```python
from build123d import *

# Parameters (mm, degrees)
F0_R     = 1.85
F0_R_2   = 4
F0_W     = 10.16
F0_H     = 6.35
F0_W_2   = 12.7
F0_W_3   = 6.35
F0_H_2   = 15.24
F0_H_3   = 8.021719
F1_DEPTH = 6.35


with BuildPart() as f1:
    # F0 (on Top) → F1 (new body)
    with BuildSketch(Plane.XY):
        with BuildLine():
            Line((-60.850162, -6.604), (-60.850162, 0))
            Line((-60.850162, 0), (-54.533258, 0))
            Line((-54.533258, 0), (-54.533258, 203.2))
            add(Edge.make_bspline(
                [(-54.533258, 203.2), (-23.033295, 215.9), (23.033295, 215.9), (54.533258, 203.2)],
                knots=[0, 0, 0, 0, 109.066515, 109.066515, 109.066515, 109.066515], degree=3))
            Line((54.533258, 203.2), (54.533258, 0))
            Line((54.533258, 0), (60.850162, 0))
            Line((60.850162, 0), (60.850162, -6.604))
            Line((60.850162, -6.604), (89.198314, -6.604))
            Line((89.198314, -6.604), (89.198314, 0))
            Line((89.198314, 0), (94.278314, 0))
            Line((94.278314, 0), (94.278314, 38.1))
            Line((94.278314, 38.1), (100.882314, 38.1))
            Line((100.882314, 38.1), (100.882314, 88.9))
            Line((100.882314, 88.9), (94.278314, 88.9))
            Line((94.278314, 88.9), (94.278314, 114.3))
            Line((94.278314, 114.3), (100.882314, 114.3))
            Line((100.882314, 114.3), (100.882314, 165.1))
            Line((100.882314, 165.1), (94.278314, 165.1))
            Line((94.278314, 165.1), (94.278314, 203.2))
            Line((94.278314, 203.2), (58.854451, 279.166719))
            Line((58.854451, 279.166719), (9.525, 279.166719))
            Line((9.525, 279.166719), (9.525, 263.525))
            Line((9.525, 263.525), (20.955, 263.525))
            Line((20.955, 263.525), (20.955, 248.285))
            Line((20.955, 248.285), (9.525, 248.285))
            Line((9.525, 248.285), (9.525, 241.066719))
            Line((9.525, 241.066719), (-9.525, 241.066719))
            Line((-9.525, 241.066719), (-9.525, 279.166719))
            Line((-9.525, 279.166719), (-58.854451, 279.166719))
            Line((-58.854451, 279.166719), (-94.278314, 203.2))
            Line((-94.278314, 203.2), (-94.278314, 165.1))
            Line((-94.278314, 165.1), (-100.882314, 165.1))
            Line((-100.882314, 165.1), (-100.882314, 114.3))
            Line((-100.882314, 114.3), (-94.278314, 114.3))
            Line((-94.278314, 114.3), (-94.278314, 88.9))
            Line((-94.278314, 88.9), (-100.882314, 88.9))
            Line((-100.882314, 88.9), (-100.882314, 38.1))
            Line((-100.882314, 38.1), (-94.278314, 38.1))
            Line((-94.278314, 38.1), (-94.278314, 0))
            Line((-94.278314, 0), (-89.198314, 0))
            Line((-89.198314, 0), (-89.198314, -6.604))
            Line((-89.198314, -6.604), (-60.850162, -6.604))
        make_face()
        with Locations((-80.681092, 9.743146)):
            Circle(F0_R, mode=Mode.SUBTRACT)
        with Locations((-80.681092, 21.056854)):
            Circle(F0_R, mode=Mode.SUBTRACT)
        with Locations((-69.367384, 9.743146)):
            Circle(F0_R, mode=Mode.SUBTRACT)
        with Locations((-75.024238, 15.4)):
            Circle(F0_R_2, mode=Mode.SUBTRACT)
        with Locations((-69.367384, 21.056854)):
            Circle(F0_R, mode=Mode.SUBTRACT)
        with Locations((-75.024238, 63.5)):
            Rectangle(F0_W, F0_H, mode=Mode.SUBTRACT)
        with Locations((69.367384, 9.743146)):
            Circle(F0_R, mode=Mode.SUBTRACT)
        with Locations((75.024238, 15.4)):
            Circle(F0_R_2, mode=Mode.SUBTRACT)
        with Locations((69.367384, 21.056854)):
            Circle(F0_R, mode=Mode.SUBTRACT)
        with Locations((80.681092, 9.743146)):
            Circle(F0_R, mode=Mode.SUBTRACT)
        with Locations((80.681092, 21.056854)):
            Circle(F0_R, mode=Mode.SUBTRACT)
        with Locations((75.024238, 63.5)):
            Rectangle(F0_W, F0_H, mode=Mode.SUBTRACT)
        with Locations((-75.024238, 139.7)):
            Rectangle(F0_W, F0_H, mode=Mode.SUBTRACT)
        with Locations((-74.405786, 200.025)):
            Rectangle(F0_W_2, F0_H, mode=Mode.SUBTRACT)
        with Locations((-17.78, 227.960319)):
            Rectangle(F0_W_3, F0_H_2, mode=Mode.SUBTRACT)
        with Locations((-17.78, 255.905)):
            Rectangle(F0_W_3, F0_H_2, mode=Mode.SUBTRACT)
        with Locations((75.024238, 139.7)):
            Rectangle(F0_W, F0_H, mode=Mode.SUBTRACT)
        with Locations((74.405786, 200.025)):
            Rectangle(F0_W_2, F0_H, mode=Mode.SUBTRACT)
        with Locations((0, 226.895859)):
            Rectangle(F0_W_3, F0_H_3, mode=Mode.SUBTRACT)
        with Locations((17.78, 227.960319)):
            Rectangle(F0_W_3, F0_H_2, mode=Mode.SUBTRACT)
    extrude(amount=F1_DEPTH)


solid = f1.part
```
Input: part model. Units: mm. Frame: model coordinates. A direction names the side the tool comes from. Round coordinates to 2 decimals unless told otherwise and drop trailing zeros. Order: outer loops, then holes, each group sorted by start corner. A loop starts at its lowest first (then second) coordinate and runs counter-clockwise, first axis right, second up. Notation, with made-up numbers: (18, 68) - (62, 68) arc R21 ccw to (62, 95) - close; hole circle Ø1 at (14, 18). An arc over 180 degrees is marked (long way). Answer in a Markdown table with one row per item.
Item 1: Section query B-B (y = 15.4). Return the cut outline in (x, z), then the cut area to 3 significant figures.
Model answer:
| item | result |
|---|---|
| outline | (-94.28, 0) - (-79.02, 0) - (-79.02, 6.35) - (-94.28, 6.35) - close; (-71.02, 0) - (-54.53, 0) - (-54.53, 6.35) - (-71.02, 6.35) - close; (54.53, 0) - (71.02, 0) - (71.02, 6.35) - (54.53, 6.35) - close; (79.02, 0) - (94.28, 0) - (94.28, 6.35) - (79.02, 6.35) - close |
| area | 403 mm² |
Item 2: Section query A-A (y = 105). Return the cut outline in (x, z).
Model answer:
| item | result |
|---|---|
| outline | (-94.28, 0) - (-54.53, 0) - (-54.53, 6.35) - (-94.28, 6.35) - close; (54.53, 0) - (94.28, 0) - (94.28, 6.35) - (54.53, 6.35) - close |
Item 3: Section query C-C (y = 149.5). Return the cut outline in (x, z).
Model answer:
| item | result |
|---|---|
| outline | (-100.88, 0) - (-54.53, 0) - (-54.53, 6.35) - (-100.88, 6.35) - close; (54.53, 0) - (100.88, 0) - (100.88, 6.35) - (54.53, 6.35) - close |
Item 4: Reachability of faces 4 (the flat face through (89.198, -3, 3)), 5 (the flat face through (75, 60.325, 3)), 6 (the flat face through (60.85, -3, 3)), 7 (the flat face through (9.525, 271, 3)), 8 (the flat face through (-98, 38.1, 3)) from +Z, -Z, +X, -X, +Y, -Y: full face, straight path, thin tool, end or side. Return the list, or none.
Model answer:
| item | result |
|---|---|
| face 4 | +Z, -Z, +X, -Y |
| face 5 | +Z, -Z |
| face 6 | +Z, -Z, -Y |
| face 7 | +Z, -Z, +Y |
| face 8 | +Z, -Z, -X, -Y |
Item 5: Mould query, pull axis Y, two halves, no side actions, for faces 1 (the flat face through (94.278, 19, 3)), 2 (the flat face through (-58, 0, 3)), 3 (the flat face through (-98, 114.3, 3)). Classes: released by +Y, released by -Y, zero draft, split by the parting line, or undercut.
Model answer:
| item | result |
|---|---|
| face 1 | zero draft |
| face 2 | released by -Y |
| face 3 | undercut |
Item 6: Section query D-D (z = 1). Give the number of separate pieces and of enclosed holes in the cut face, then the cut area to 3 significant figures.
Model answer:
| item | result |
|---|---|
| separate pieces | 1 |
| enclosed holes | 20 |
| area | 26,900 mm² |
Item 7: Pin query (flat end, axial travel): pin 1 (3 mm diameter, centred on x = 98, z = 4, fed in from -Y); pin 2 (1 mm diameter, centred on y = 167, z = 3.5, fed in from -X); pin 3 (1.9 mm diameter, centred on x = -98, z = 3.5, fed in from +Y). Return the tip coordinate at first contact, or that it passes through.
Model answer:
| item | result |
|---|---|
| pin 1 | stops at y = 38.1 |
| pin 2 | stops at x = -94.28 |
| pin 3 | stops at y = 165.1 |
Item 8: Line query: line 1 (X direction, y = 100, z = 3.75); line 2 (X direction, y = 118.5, z = 4.5); line 3 (X direction, y = 228.5, z = 1.75) (3 decimals). Output: solid intervals per line, ascending.
Model answer:
| item | result |
|---|---|
| line 1 | x = -94.28 to -54.53, 54.53 to 94.28 |
| line 2 | x = -100.88 to -54.53, 54.53 to 100.88 |
| line 3 | x = -82.481 to -20.955, -14.605 to -3.175, 3.175 to 14.605, 20.955 to 82.481 |
